Autodesk Inventor part; units mm, degrees
ref_plane "Work Plane1" through (30.1625, 0, 0) normal (0, 0, -1) x (1, 0, 0)
ref_plane "YZ Plane" through (0, 0, 0) normal (1, 0, 0) x (0, 1, 0)
ref_plane "XZ Plane" through (0, 0, 0) normal (0, 1, 0) x (-1, 0, 0)
sketch "Эскиз1" plane through (0, 0, 0) normal (0, 0, 1) x (1, 0, 0)
  line L0 (-6, 0) -> (18, 0)
  line L1 (18, 0) -> (18, 5)
  line L2 (18, 5) -> (1.5, 5)
  line L3 (1.5, 5) -> (0.5798, 5)
  line L4 (0.5798, 5) -> (0, 5)
  line L5 (0, 5) -> (0, 8)
  line L6 (-10.8, 0) -> (22.8, 0)
  line L7 (0, -1.6) -> (0, 9.6)
  line L8 (-6, 0) -> (-6, 8)
  line L9 (0, 8) -> (-6, 8)
  dimension "d0" = 18
  dimension "d1" = 16.5
  dimension "d2" = 0.9202
  dimension "d3" = 6
  dimension "d4" = 10
  dimension "d5" = 10
  dimension "d9" = 16
  dimension "d10" = 0
revolve "Базовый элемент" add sketch "Эскиз1" angle 360 about axis through (-6, 0, 0) along (1, 0, 0)
sketch "Эскиз2" plane through (-6, 0, 0) normal (-1, 0, 0) x (0, 0, 1)
  circle A0 centre (0, 0) radius 8
  line L0 (0, 0) -> (0, 8)
  line L1 (-8, 1.05) -> (8, 1.05)
  line L2 (8, 1.05) -> (8, -1.05)
  line L3 (8, -1.05) -> (-8, -1.05)
  line L4 (-8, -1.05) -> (-8, 1.05)
  line L5 (-8, 0) -> (8, 0) construction
  line L6 (0, 1.05) -> (0, -1.05) construction
  dimension "d11" = 2.1
  dimension "d12" = 16
fillet "Сопряжение1" radius 0.01 1 edges at (-6, -8, 0)
extrude "Паз" cut sketch "Эскиз2" against normal blind 4.2 contours A0 L3 L1 | L2 L3 A0 | A0 L1 L2 | L3 L4 A0 | A0 L4 L1
thread "Резьба"
chamfer "Chamfer4" distance 1 angle 45 1 edges at (18, -5, 0)
ref_plane "Work Plane1" through (30.1625, 0, 0) normal (0, 0, -1) x (1, 0, 0)
equation "\"d11\" = SBR"
equation "\"d12\" = KOD"
equation "\"d13\" = RR"
equation "\"d16\" = STI"
equation "\"d14\" = GEL"
equation "\"d40\" = 0.1 * GD"
equation "\"d0\" = NLG"
equation "\"d1\" = GEL"
equation "\"d2\" = GAL"
equation "\"d3\" = KOH"
equation "\"d4\" = GD"
equation "\"d5\" = BDM"
equation "\"d9\" = KOD"
equation "\"GD\" = NND"
equation "\"NLG\" = 18"
equation "\"GEL\" = 16.5"
equation "\"KOD\" = 16"
equation "\"KOH\" = 6"
equation "\"GAL\" = 0.61345 * PTC"
equation "\"BDM\" = NND"
equation "\"RR\" = 0.01"
equation "\"SBR\" = 2.1"
equation "\"STI\" = 4.2"
equation "\"KEWI\" = 0"
equation "\"GUL\" = 0.61345 * PTC"
equation "\"SPD\" = NND - 1.2269 * PTC"
equation "\"PTC\" = 1.5"
equation "\"TOA\" = 30deg"
equation "\"FAWI\" = 45deg"
equation "\"GD1\" = THREADDIA - 1.2269 * PTC"
properties part number "Винт M10-6gx18 ГОСТ 1491-80" material "Сталь, мягкая"
Can you work these out from the model? Positions are in its coordinate system, mm. A direction names the side the tool comes from. Give positions to 0.01 mm unless a question says otherwise; leave off trailing zeros. Order: outer loops, then holes, each group sorted by start corner. A loop starts at its lowest first (then second) coordinate and runs counter-clockwise, first axis right, second up. Notation, with made-up numbers: M 25.25,31.25 L 49.25,31.25 A20 cw 49.25,60.25 Z; hole C -37.5,-3.75 d8. An arc over 180 degrees is marked long. Use one line per item in the form item = value. Start each with the question number.
Item 1: For faces 1 (the flat face through (-6, -4, 0)), 2 (the cylindrical face through (8.38, -1.08, 4.88)), 3 (the flat face through (-1.8, 0, 0)), which set-ups out of +Z, -Z, +X, -X, +Y, -Y let a thin tool reach every point of the face, with its end or its side?
Item 2: We'd pull the mould along Y, two halves only. Please class faces 4 (the cylindrical face through (-3.04, -1.73, 7.81)), 5 (the flat face through (-6, 4, 0)), 6 (the flat face through (-4, 1.05, 0)): +Y half, -Y half, draft (parallel to the pull), parting line (faces both ways), or undercut.
Item 3: If I drill on line 1 along Y through (x, z) = (-2.25, -0.25); line 2 along Y through (x, z) = (1.5, -0.25); line 3 along X through (y, z) = (-1.5, -7.5), over which ranges is the centre line in solid material (lowest first)?
Item 4: Will these pins go through, and if not, where does the flat tip stop? pin 1 Ø6 at (x, z) = (14, 5) entering from -Y; pin 2 Ø8 at (x, y) = (13.5, -1) entering from +Z; pin 3 Ø2 at (x, y) = (12, -5) entering from -Z.
Item 5: If we section it at C-C (x = 6.75): Write out the boundary of the cut face in (y, z).
Item 6: If we section it at A-A (y = 0): Write out the boundary of the cut face in (x, z), then the cut area to 3 significant figures.
Outcome:
q1.face_1 = +Z, -Z, -X, +Y, -Y
q1.face_2 = +X
q1.face_3 = +Z, -Z, -X
q2.face_4 = parting line
q2.face_5 = draft
q2.face_6 = undercut
q3.line_1 = -8 to -1.05, 1.05 to 8
q3.line_2 = -4.99 to 4.99
q3.line_3 = -6 to 0
q4.pin_1 = -4.58
q4.pin_2 = 5
q4.pin_3 = -3
q5.outline = C 0,0 d10
q6.outline = M -1.8,-8 L 0,-8 L 0,-5 L 17,-5 L 18,-4 L 18,4 L 17,5 L 0,5 L 0,8 L -1.8,8 Z
q6.area = 208 mm2
